from build123d import *

# Parameters (mm, degrees)
ESQUISSE1_W             = 130
ESQUISSE1_H             = 190
BOSS_EXTRU_1_DEPTH      = 6
ENL_V_MAT_EXTRU_1_DEPTH = 125.342269563
ESQUISSE3_R             = 2.19
ESQUISSE3_W             = 15
ESQUISSE3_H             = 2.95
ENL_V_MAT_EXTRU_2_DEPTH = 125.342269563
ESQUISSE5_R             = 3
ENL_V_MAT_EXTRU_3_DEPTH = 125.342269563
CUT_EXTRUDE1_REACH      = 126.342
SKETCH1_W               = 22.17
SKETCH1_H               = 41.26
FILLET1_R               = 1
M4_CLEARANCE_HOLE1_D    = 4.5
CUT_EXTRUDE2_REACH      = 126.342
SKETCH5_W               = 15
SKETCH5_H               = 82.5
FILLET2_R               = 25
FILLET3_R               = 3
F_8_CLEARANCE_HOLE1_D   = 4.4958


with BuildPart() as part:
    # Esquisse1 → Boss.-Extru.1 (new body)
    with BuildSketch(Plane(origin=(0, 0, 0), x_dir=(1, 0, 0), z_dir=(0, 1, 0))):
        with Locations((-15, 0)):
            Rectangle(ESQUISSE1_W, ESQUISSE1_H)
    extrude(amount=-BOSS_EXTRU_1_DEPTH)

    # Esquisse2 → Enlèv. mat.-Extru.1 (cut, through all)
    with BuildSketch(Plane.XZ.offset(6)):
        with BuildLine():
            Line((-6.35, 75), (-6.35, 50))
            ThreePointArc((-6.35, 50), (0, 43.65), (6.35, 50))
            Line((6.35, 50), (6.35, 75))
            ThreePointArc((6.35, 75), (0, 81.35), (-6.35, 75))
        make_face()
        with BuildLine():
            Line((15.258, 88.470384182), (15.258, 36.529615818))
            ThreePointArc((15.258, 36.529615818), (13.48, 34.751615818), (11.702, 36.529615818))
            Line((11.702, 36.529615818), (11.702, 88.470384182))
            ThreePointArc((11.702, 88.470384182), (13.48, 90.248384182), (15.258, 88.470384182))
        make_face()
        with BuildLine():
            Line((-15.258, 88.470384182), (-15.258, 36.529615818))
            ThreePointArc((-15.258, 36.529615818), (-13.48, 34.751615818), (-11.702, 36.529615818))
            Line((-11.702, 36.529615818), (-11.702, 88.470384182))
            ThreePointArc((-11.702, 88.470384182), (-13.48, 90.248384182), (-15.258, 88.470384182))
        make_face()
        with BuildLine():
            Line((15.258, -88.470384182), (15.258, -36.529615818))
            ThreePointArc((15.258, -36.529615818), (13.48, -34.751615818), (11.702, -36.529615818))
            Line((11.702, -36.529615818), (11.702, -88.470384182))
            ThreePointArc((11.702, -88.470384182), (13.48, -90.248384182), (15.258, -88.470384182))
        make_face()
        with BuildLine():
            Line((-6.35, -75), (-6.35, -50))
            ThreePointArc((-6.35, -50), (0, -43.65), (6.35, -50))
            Line((6.35, -50), (6.35, -75))
            ThreePointArc((6.35, -75), (0, -81.35), (-6.35, -75))
        make_face()
        with BuildLine():
            Line((-15.258, -88.470384182), (-15.258, -36.529615818))
            ThreePointArc((-15.258, -36.529615818), (-13.48, -34.751615818), (-11.702, -36.529615818))
            Line((-11.702, -36.529615818), (-11.702, -88.470384182))
            ThreePointArc((-11.702, -88.470384182), (-13.48, -90.248384182), (-15.258, -88.470384182))
        make_face()
    extrude(amount=-ENL_V_MAT_EXTRU_1_DEPTH, mode=Mode.SUBTRACT)

    # Esquisse3 → Enlèv. mat.-Extru.2 (cut, through all)
    with BuildSketch(Plane.XZ.offset(6)):
        with Locations(Location((-53.085, -9.02, 0), (0, 0, 270))):
            Circle(ESQUISSE3_R)
        with Locations(Location((-42.915, -56.28, 0), (0, 0, 270))):
            Circle(ESQUISSE3_R)
        with Locations(Location((-53.085, -56.28, 0), (0, 0, 270))):
            Circle(ESQUISSE3_R)
        with Locations(Location((-42.915, -9.02, 0), (0, 0, 270))):
            Circle(ESQUISSE3_R)
        with Locations((-32.5, 3.975)):
            Rectangle(ESQUISSE3_W, ESQUISSE3_H)
        with Locations((22.5, 3.975)):
            Rectangle(ESQUISSE3_W, ESQUISSE3_H)
        with Locations((22.5, -3.975)):
            Rectangle(ESQUISSE3_W, ESQUISSE3_H)
        with Locations((-32.5, -3.975)):
            Rectangle(ESQUISSE3_W, ESQUISSE3_H)
    extrude(amount=-ENL_V_MAT_EXTRU_2_DEPTH, mode=Mode.SUBTRACT)

    # Esquisse5 → Enlèv. mat.-Extru.3 (cut, through all)
    with BuildSketch(Plane.XZ.offset(6)):
        with Locations(Location((-28, 23, 0), (0, 0, 270))):
            Circle(ESQUISSE5_R)
        with Locations(Location((-28, -23, 0), (0, 0, 270))):
            Circle(ESQUISSE5_R)
    extrude(amount=-ENL_V_MAT_EXTRU_3_DEPTH, mode=Mode.SUBTRACT)

    # Sketch1 → Cut-Extrude1 (cut, up to next)
    with BuildSketch(Plane.XZ.offset(6), mode=Mode.PRIVATE) as cut_extrude1_sk1:
        with Locations((-48, -32.65)):
            Rectangle(SKETCH1_W, SKETCH1_H)
    cut_extrude1_tool1 = extrude(cut_extrude1_sk1.sketch, amount=-CUT_EXTRUDE1_REACH, mode=Mode.PRIVATE) & part.part
    add(cut_extrude1_tool1.solids().sort_by_distance((-48, -6, -32.65))[0], mode=Mode.SUBTRACT)

    # Fillet1
    fillet1_edges = [part.edges().sort_by_distance(p)[0] for p in [
        (-59.085, -3, -53.28),
        (-59.085, -3, -12.02),
        (-36.915, -3, -12.02),
        (-36.915, -3, -53.28),
    ]]
    fillet(fillet1_edges, radius=FILLET1_R)

    # M4 Clearance Hole1 (through all)
    with Locations(Plane(origin=(0, -6, 0), x_dir=(-1, 0, 0), z_dir=(0, -1, 0))):
        with Locations((-28, -45.2375), (-44, -60), (28, -45.2375), (44, -60), (60, -45.2375)):
            Hole(M4_CLEARANCE_HOLE1_D / 2)

    # Sketch5 → Cut-Extrude2 (cut, up to next)
    with BuildSketch(Plane.XZ.offset(6), mode=Mode.PRIVATE) as cut_extrude2_sk1:
        with Locations((-72.5, 53.75)):
            Rectangle(SKETCH5_W, SKETCH5_H)
    cut_extrude2_tool1 = extrude(cut_extrude2_sk1.sketch, amount=-CUT_EXTRUDE2_REACH, mode=Mode.PRIVATE) & part.part
    # Sketch5 → Cut-Extrude2 (cut, up to next)
    with BuildSketch(Plane.XZ.offset(6), mode=Mode.PRIVATE) as cut_extrude2_sk2:
        with Locations((-72.5, -53.75)):
            Rectangle(SKETCH5_W, SKETCH5_H)
    cut_extrude2_tool2 = extrude(cut_extrude2_sk2.sketch, amount=-CUT_EXTRUDE2_REACH, mode=Mode.PRIVATE) & part.part
    add(cut_extrude2_tool1.solids().sort_by_distance((-72.5, -6, 53.75))[0], mode=Mode.SUBTRACT)
    add(cut_extrude2_tool2.solids().sort_by_distance((-72.5, -6, -53.75))[0], mode=Mode.SUBTRACT)

    # Fillet2
    fillet2_edges = [part.edges().sort_by_distance(p)[0] for p in [
        (-65, -3, 95),
        (-65, -3, -95),
        (50, -3, -95),
        (50, -3, 95),
    ]]
    fillet(fillet2_edges, radius=FILLET2_R)

    # Fillet3
    fillet3_edges = [part.edges().sort_by_distance(p)[0] for p in [
        (-65, -3, 12.5),
        (-80, -3, 12.5),
        (-80, -3, -12.5),
        (-65, -3, -12.5),
    ]]
    fillet(fillet3_edges, radius=FILLET3_R)

    # #8 Clearance Hole1 (through all)
    with Locations(Plane(origin=(0, 0, 0), x_dir=(1, 0, 0), z_dir=(0, 1, 0))):
        with Locations((16.3, 11.394380081), (-17.7, 11.394380081), (44.3, 11.394380081)):
            Hole(F_8_CLEARANCE_HOLE1_D / 2)


solid = part.part
Source: CAD feature listing. Evaluate the final solid. Frame: model axes, mm. A direction names the side the tool comes from. Give positions to 0.01 mm unless a question says otherwise; leave off trailing zeros. Loops run counter-clockwise (first coordinate to the right, second up) from the corner with the lowest first, then second, coordinate; pieces in that order, holes last. Notation, with made-up numbers: (73.5, 85) -> (109.5, 85) arc R30 cw to (109.5, 120) -> close; hole circle Ø6 at (58, 1). An arc over 180 degrees is marked (long way). Use a Markdown table: item, result. Add a question column.
1) First-contact query: pin 1 (3 mm diameter, centred on x = -46.5, y = -5, fed in from -Z); pin 2 (6 mm diameter, centred on x = -39.5, z = -16, fed in from -Y); pin 3 (3 mm diameter, centred on y = -3, z = -50, fed in from -X); pin 4 (3.5 mm diameter, centred on x = -53.085, z = -9.02, fed in from -Y). Flat tips, straight axial feed; report the tip coordinate or a pass-through.
2) Reachability of faces 1 (the face through (-16, 0, -1)), 2 (the face through (-59.085, -3, -33)) from +Z, -Z, +X, -X, +Y, -Y: full face, straight path, thin tool, end or side. Return the list, or none.
3) Section query C-C, the plane x = 44.3. Return the cut outline in (y, z), then the cut area to 3 significant figures.
4) Pull-direction query (Z, two-part tool) for faces 3 (the face through (42.214, -2.958, 61.369)), 4 (the face through (42.871, -3.042, 87.482)), 5 (the face through (-73, -3, -12.5)); classes: +Z half, -Z half, draft (parallel to the pull), parting line (faces both ways), or undercut.
5) Section query D-D, the plane y = -4.9. Count the separate pieces of the cut face and the enclosed holes in it, then the cut area to 3 significant figures.
6) Section query A-A, the plane z = 60. Return the cut outline in (x, y).
7) Line query: line 1 along X through (y, z) = (-4.15, -66); line 2 along X through (y, z) = (-2.95, -40) (3 decimals); line 3 along X through (y, z) = (-4.5, 23). Output: solid intervals per line, ascending. Write a range as [from, to].
8) Section query B-B, the plane x = 23. Return the cut outline in (y, z), then the cut area to 3 significant figures.
Numbers:
| question | item | result |
|---|---|---|
| 1 | pin 1 | stops at z = -94.49 |
| 1 | pin 2 | stops at y = -6 |
| 1 | pin 3 | stops at x = -65 |
| 1 | pin 4 | passes through |
| 2 | face 1 | +Z, -Z, +X, -X, +Y |
| 2 | face 2 | +Y, -Y |
| 3 | outline | (-6, -85.89) -> (0, -85.89) -> (0, -13.64) -> (-6, -13.64) -> close; (-6, -9.15) -> (0, -9.15) -> (0, 57.77) -> (-6, 57.77) -> close; (-6, 62.23) -> (0, 62.23) -> (0, 85.89) -> (-6, 85.89) -> close |
| 3 | area | 977 mm2 |
| 4 | face 3 | undercut |
| 4 | face 4 | +Z half |
| 4 | face 5 | -Z half |
| 5 | separate pieces | 1 |
| 5 | enclosed holes | 25 |
| 5 | area | 18,700 mm2 |
| 6 | outline | (-65, -6) -> (-46.25, -6) -> (-46.25, 0) -> (-65, 0) -> close; (-41.75, -6) -> (-15.26, -6) -> (-15.26, 0) -> (-41.75, 0) -> close; (-11.7, -6) -> (-6.35, -6) -> (-6.35, 0) -> (-11.7, 0) -> close; (6.35, -6) -> (11.7, -6) -> (11.7, 0) -> (6.35, 0) -> close; (15.26, -6) -> (41.75, -6) -> (41.75, 0) -> (15.26, 0) -> close; (46.25, -6) -> (50, -6) -> (50, 0) -> (46.25, 0) -> close |
| 7 | line 1 | x = [-65, -15.26], [-11.7, -6.35], [6.35, 11.7], [15.26, 50] |
| 7 | line 2 | x = [-65, -59.085], [-36.915, -15.258], [-11.702, 11.702], [15.258, 50] |
| 7 | line 3 | x = [-65, -31], [-25, 50] |
| 8 | outline | (-6, -95) -> (0, -95) -> (0, -5.45) -> (-6, -5.45) -> close; (-6, -2.5) -> (0, -2.5) -> (0, 2.5) -> (-6, 2.5) -> close; (-6, 5.45) -> (0, 5.45) -> (0, 95) -> (-6, 95) -> close |
| 8 | area | 1,100 mm2 |
